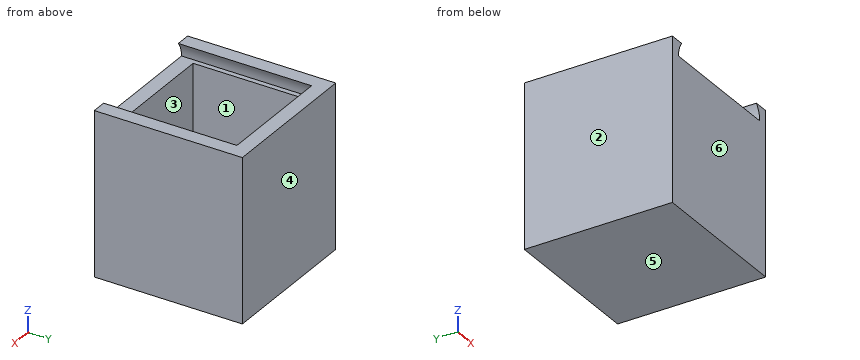
```python
from build123d import *

# Parameters (mm, degrees)
F0_W     = 25.4
F0_H     = 27.94
F1_DEPTH = 25.4
F2_T     = -2.54
F4_DEPTH = 22.86


with BuildPart() as f1:
    # F0 (on Front) → F1 (new body)
    with BuildSketch(Plane.XZ):
        Rectangle(F0_W, F0_H)
    extrude(amount=F1_DEPTH)

    # F2
    f2_openings = [f1.faces().sort_by_distance(p)[0] for p in [
        (0, -12.7, 13.97),
    ]]
    offset(amount=F2_T, openings=f2_openings)

    # F3 (on face) → F4 (cut)
    with BuildSketch(Plane.XZ.offset(25.4)):
        with BuildLine():
            Line((-11.049, 11.43), (11.061186, 11.43))
            ThreePointArc((11.061186, 11.43), (10.829213, 12.777566), (10.16, 13.97))
            Line((10.16, 13.97), (-10.16, 13.97))
            ThreePointArc((-10.16, 13.97), (-10.820331, 12.775541), (-11.049, 11.43))
        make_face()
    extrude(amount=-F4_DEPTH, mode=Mode.SUBTRACT)


solid = f1.part
```
The listing builds one solid part. Answer for the finished solid, in the listing's coordinates (mm). Face numbers are marked on the shaded views. A direction names the side the tool comes from. Round coordinates to 2 decimals unless told otherwise and drop trailing zeros. Loops run counter-clockwise (first coordinate to the right, second up) from the corner with the lowest first, then second, coordinate; pieces in that order, holes last. Notation, with made-up numbers: (48.5, -24.75) - (52.5, -24.75) arc R27 ccw to (52.5, 13.25) - close; hole circle Ø6 at (59, -0.75). An arc over 180 degrees is marked (long way). Use one line per item in the form item = value. Start each with the question number.
1. The part is cut by section D-D on y = -11.75. Determine the outline of the cut face in (x, z), then the cut area to 3 significant figures.
2. A tool of negligible diameter and unlimited length cuts with its end or side. For the marked faces 1 and 2, from which of +Z, -Z, +X, -X, +Y, -Y can it reach the whole face along a straight path? Write none if from no direction.
3. Consider line 1 (Y direction, x = 3.75, z = -9); line 2 (X direction, y = -15, z = -4); line 3 (X direction, y = -5.75, z = 11.5). Determine where each line is inside the solid, lowest interval first. Write a range as [from, to].
4. The part is cut by section A-A on z = 0.75. Determine the outline of the cut face in (x, y), then the cut area to 3 significant figures.
5. The part is cut by section B-B on x = 5.25. Determine the outline of the cut face in (y, z).
6. For a pull along Y with two mould halves and no side action, classify the marked faces 3, 4, 5 and 6 as pulls with the +Y half, pulls with the -Y half, needs draft (parallel to the pull), parting line crosses it, or undercut.
7. The part is cut by section C-C on y = -23.5. Determine the outline of the cut face in (x, z), then the cut area to 3 significant figures.
Geometry check:
q1.outline = (-12.7, -13.97) - (12.7, -13.97) - (12.7, 13.97) - (10.16, 13.97) arc R4.03 cw to (11.06, 11.43) - (10.16, 11.43) - (10.16, -11.43) - (-10.16, -11.43) - (-10.16, 11.43) - (-11.05, 11.43) arc R4.07 cw to (-10.16, 13.97) - (-12.7, 13.97) - close
q1.area = 190 mm^2
q2.face_1 = +Z
q2.face_2 = +Z, -Z, -X, +Y, -Y
q3.line_1 = [-25.4, -22.86], [-2.54, 0]
q3.line_2 = [-12.7, -10.16], [10.16, 12.7]
q3.line_3 = [-12.7, -11.05], [11.06, 12.7]
q4.outline = (-12.7, -25.4) - (12.7, -25.4) - (12.7, 0) - (-12.7, 0) - close; hole (-10.16, -22.86) - (10.16, -22.86) - (10.16, -2.54) - (-10.16, -2.54) - close
q4.area = 232 mm^2
q5.outline = (-25.4, -13.97) - (0, -13.97) - (0, 13.97) - (-2.54, 13.97) - (-2.54, -11.43) - (-22.86, -11.43) - (-22.86, 11.43) - (-25.4, 11.43) - close
q6.face_3 = undercut
q6.face_4 = pulls with the +Y half
q6.face_5 = needs draft
q6.face_6 = pulls with the -Y half
q7.outline = (-12.7, -13.97) - (12.7, -13.97) - (12.7, 13.97) - (10.16, 13.97) arc R4.03 cw to (11.06, 11.43) - (-11.05, 11.43) arc R4.07 cw to (-10.16, 13.97) - (-12.7, 13.97) - close
q7.area = 655 mm^2
